```python
from build123d import *

# Parameters (mm, degrees)
BOSS_EXTRUDE1_DEPTH  = 2
SKETCH12_R           = 25
BOSS_EXTRUDE2_DEPTH  = 8
CUT_EXTRUDE6_START   = -36
SKETCH17_R           = 10.33
CUT_EXTRUDE6_DEPTH   = 45.856111051
SKETCH25_R           = 30
BOSS_EXTRUDE3_DEPTH  = 5
CUT_EXTRUDE9_START   = -53
SKETCH26_R           = 10.33
CUT_EXTRUDE9_DEPTH   = 53
FILLET3_R            = 1.5
SKETCH23_R           = 7.75
CUT_EXTRUDE11_DEPTH  = 36
FILLET3_OF_MIRROR1_R = 1.5
CUT_EXTRUDE12_START  = -10
SKETCH28_R           = 10.33
CUT_EXTRUDE12_DEPTH  = 10


with BuildPart() as part:
    # Sketch3 → Boss-Extrude1 (new body)
    with BuildSketch(Plane(origin=(0, 0, 0), x_dir=(1, 0, 0), z_dir=(0, 1, 0))):
        Polygon((35.1, 0), (24.81944802, 24.81944802), (0, 35.1), (-24.81944802, 24.81944802), (-35.1, 0), (-24.81944802, -24.81944802), (0, -35.1), (24.81944802, -24.81944802), align=None)
    boss_extrude1 = extrude(amount=BOSS_EXTRUDE1_DEPTH)

    # Sketch12 → Boss-Extrude2 (add)
    with BuildSketch(Plane(origin=(0, 2, 0), x_dir=(1, 0, 0), z_dir=(0, 1, 0))):
        with Locations(Location((0, 0, 0), (0, 0, 270))):
            Circle(SKETCH12_R)
    boss_extrude2 = extrude(amount=BOSS_EXTRUDE2_DEPTH)

    # Sketch17 → Cut-Extrude6 (cut)
    with BuildSketch(Plane(origin=(0, 10, 0), x_dir=(1, 0, 0), z_dir=(0, 1, 0)).offset(CUT_EXTRUDE6_START)):
        with Locations(Location((0, 7, 0), (0, 0, 270))):
            Circle(SKETCH17_R)
    cut_extrude6 = extrude(amount=CUT_EXTRUDE6_DEPTH, mode=Mode.SUBTRACT)

    # Sketch25 → Boss-Extrude3 (add)
    with BuildSketch(Plane(origin=(0, 10, 0), x_dir=(1, 0, 0), z_dir=(0, 1, 0))):
        with Locations(Location((0, 0, 0), (0, 0, 270))):
            Circle(SKETCH25_R)
    boss_extrude3 = extrude(amount=BOSS_EXTRUDE3_DEPTH)

    # Sketch26 → Cut-Extrude9 (cut)
    with BuildSketch(Plane(origin=(0, 15, 0), x_dir=(1, 0, 0), z_dir=(0, 1, 0)).offset(CUT_EXTRUDE9_START)):
        with Locations(Location((0, 7, 0), (0, 0, 270))):
            Circle(SKETCH26_R)
    extrude(amount=CUT_EXTRUDE9_DEPTH, mode=Mode.SUBTRACT)

    # Fillet3
    fillet3_edges = [part.edges().sort_by_distance(p)[0] for p in [
        (12.40972401, 2, -29.95972401),
        (-12.40972401, 2, -29.95972401),
        (-29.95972401, 2, -12.40972401),
        (-29.95972401, 2, 12.40972401),
        (-12.40972401, 2, 29.95972401),
        (12.40972401, 2, 29.95972401),
        (29.95972401, 2, 12.40972401),
        (29.95972401, 2, -12.40972401),
    ]]
    fillet(fillet3_edges, radius=FILLET3_R)

    # Sketch23 → Cut-Extrude11 (cut, symmetric)
    with BuildSketch(Plane(origin=(0, 10, 0), x_dir=(1, 0, 0), z_dir=(0, 1, 0))):
        with Locations(Location((-10.75, -17.75, 0), (0, 0, 270))):
            Circle(SKETCH23_R)
        with Locations(Location((10.75, -17.75, 0), (0, 0, 270))):
            Circle(SKETCH23_R)
    cut_extrude11 = extrude(amount=CUT_EXTRUDE11_DEPTH, both=True, mode=Mode.SUBTRACT)

    # Mirror1: Boss-Extrude1, Boss-Extrude2, Cut-Extrude6, Boss-Extrude3, Cut-Extrude11 across plane
    add(boss_extrude1.mirror(Plane.ZX))
    add(boss_extrude2.mirror(Plane.ZX))
    add(cut_extrude6.mirror(Plane.ZX), mode=Mode.SUBTRACT)
    add(boss_extrude3.mirror(Plane.ZX))
    add(cut_extrude11.mirror(Plane.ZX), mode=Mode.SUBTRACT)

    # Fillet3 of Mirror1
    fillet3_of_mirror1_edges = [part.edges().sort_by_distance(p)[0] for p in [
        (12.40972401, -2, -29.95972401),
        (-12.40972401, -2, -29.95972401),
        (-29.95972401, -2, -12.40972401),
        (-29.95972401, -2, 12.40972401),
        (-12.40972401, -2, 29.95972401),
        (12.40972401, -2, 29.95972401),
        (29.95972401, -2, 12.40972401),
        (29.95972401, -2, -12.40972401),
    ]]
    fillet(fillet3_of_mirror1_edges, radius=FILLET3_OF_MIRROR1_R)

    # Sketch28 → Cut-Extrude12 (cut)
    with BuildSketch(Plane.XZ.offset(15).offset(CUT_EXTRUDE12_START)):
        with Locations(Location((0, -7, 0), (0, 0, 270))):
            Circle(SKETCH28_R)
    extrude(amount=CUT_EXTRUDE12_DEPTH, mode=Mode.SUBTRACT)


solid = part.part
```
Design review of the part built by this model. Coordinates are the model's own, in mm. A direction names the side the tool comes from. Round coordinates to 2 decimals unless told otherwise and drop trailing zeros. Order: outer loops, then holes, each group sorted by start corner. A loop starts at its lowest first (then second) coordinate and runs counter-clockwise, first axis right, second up. Notation, with made-up numbers: M 46,12 L 75,12 A34 ccw 75,47 Z; hole C 56.25,77.25 d6. An arc over 180 degrees is marked long. Put each result on its own line as item: value.
Q1. Consider section A-A (y = 3.75). State the section outline as (x, z) points.
Reported:
outline: M -18.45,16.87 A25 ccw long 18.45,16.87 A7.75 cw long 6.4,24.17 A25 ccw -6.4,24.17 A7.75 cw long Z; hole C 0,-7 d20.66
Q2. Consider section B-B (z = 16). State how many separate pieces and enclosed holes the cut face has, and give its area (3 significant figures).
Reported:
separate pieces: 3
enclosed holes: 0
area: 442 mm²
Q3. Draft analysis for pull direction Y (two halves, no side actions). For faces 4 (the face through (29.471, 1.572, -12.411)), 5 (the face through (-29.471, -1.572, 12.411)), 6 (the face through (-3, -2, -25)), state which applies: released by +Y, released by -Y, zero draft, split by the parting line, or undercut.
Reported:
face 4: released by +Y
face 5: released by -Y
face 6: undercut
Q4. Insertion check: pin 1 Ø5 at (x, y) = (12.5, -9.5) entering from -Z; pin 2 Ø4 at (x, y) = (28, 0.5) entering from -Z; pin 3 Ø6 at (y, z) = (-2, 4.5) entering from +X. Each pin has a flat end and moves straight along its axis. Give the tip position at first contact, or say it passes through.
Reported:
pin 1: z = -28.27
pin 2: z = -21.97
pin 3: x = 34.34
Q5. Machinability: for faces 1 (the face through (0.809, -5.944, -24.987)), 2 (the face through (29.615, -1.572, 12.063)), 3 (the face through (0, 6, 25)), which of the approach directions +Z, -Z, +X, -X, +Y, -Y give a long, thin tool a straight path to every point of the face, cutting with its end or side? Answer none if there is none.
Reported:
face 1: none
face 2: +Z, +X, -Y
face 3: +Z
Q6. Consider section C-C (y = 11.5). State the section outline as (x, z) points.
Reported:
outline: C 0,0 d60; hole C -10.75,17.75 d15.5; hole C 0,-7 d20.66; hole C 10.75,17.75 d15.5
Q7. To check wall thickness, follow line 1 (Y direction, x = -16, z = -25); line 2 (Z direction, x = 5.5, y = -12.75); line 3 (X direction, y = 10.5, z = 17.75). State the ranges of each line that lie inside material, in increasing order.
Reported:
line 1: -15 to -10, -2 to 2, 10 to 15
line 2: -29.49 to -15.74, 1.74 to 12.05, 23.45 to 29.49
line 3: -24.19 to -18.5, -3 to 3, 18.5 to 24.19
